Job drawing, mm, ordinate dimensions from the low corner. One solid piece. A direction names the side the tool comes from. Coordinates: 2 decimals unless noted, no trailing zeros. Loops run counter-clockwise (first coordinate to the right, second up) from the corner with the lowest first, then second, coordinate; pieces in that order, holes last. Notation, with made-up numbers: (54, 87.25) - (76, 87.25) arc R16 ccw to (76, 114.25) - close; hole circle Ø10 at (20, 34). An arc over 180 degrees is marked (long way). Use a Markdown table: item, result. Add a question column.
1) Probe probe 1 along Y at (x, z) = (11, 9.75); probe 2 along Z at (x, y) = (21.55, 11); probe 3 along Z at (x, y) = (14.25, 7.5). List the from-to ranges inside material, lowest first. Write a range as [from, to].
2) Band-saw the part on A-A (x = 11). Give the cut face in (y, z).
3) Band-saw the part on D-D (y = 16.75). Give the cut face in (x, z), plus the area to 3 significant figures.
4) Drop flat-ended pins along their axis: P1, Ø8, axis at x = 11, z = 8, coming from the +Y side; P2, Ø2, axis at y = 11.5, z = 4.5, coming from the +X side; P3, Ø6, axis at x = 11, y = 11, coming from the +Z side. Give the stop position or say it passes through.
5) Band-saw the part on C-C (z = 8). Give the cut face in (x, y), plus the area to 3 significant figures.
6) Tool access for the marked faces 4, 5, 6 and 7: list every direction of +Z, -Z, +X, -X, +Y, -Y with a clear straight run to the whole face (end or side of a thin tool).
7) Pull direction Z, two halves, no side cores. Call the marked faces 1, 2 and 3: +Z half, -Z half, draft (parallel to the pull), parting line (faces both ways), or undercut.
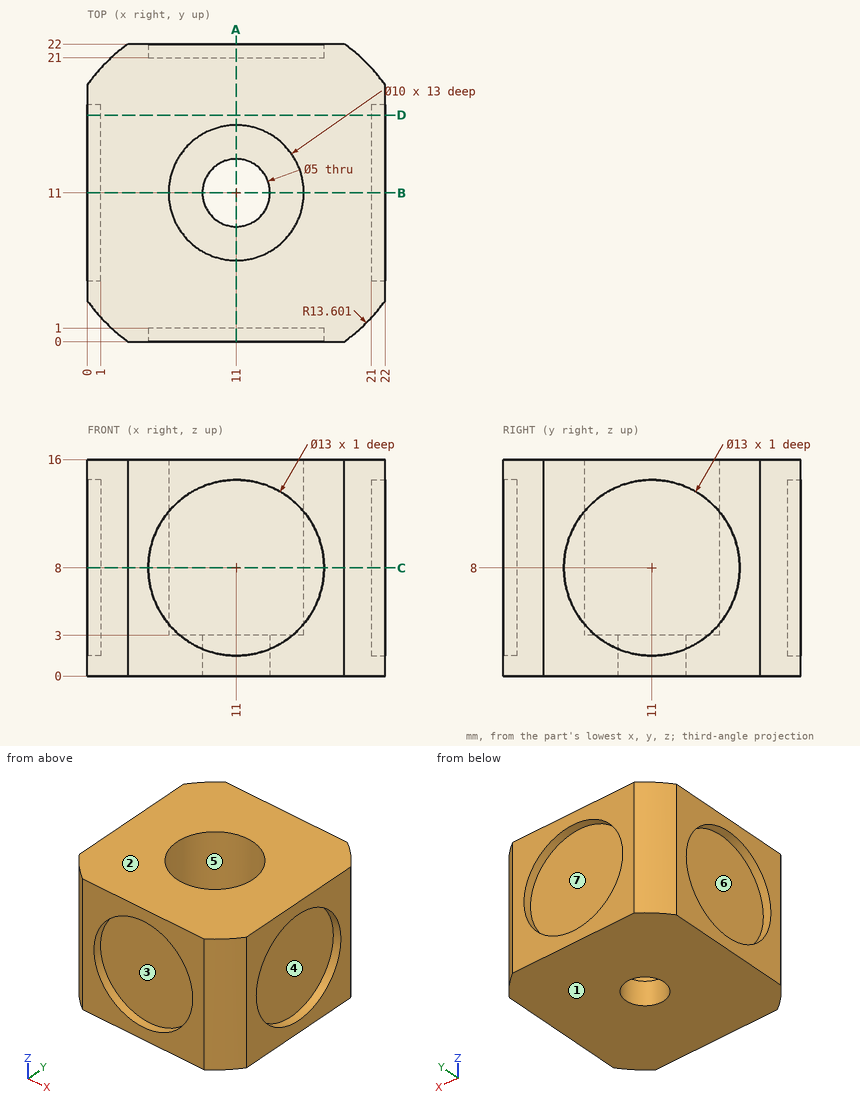
Answer block:
| question | item | result |
|---|---|---|
| 1 | probe 1 | [1, 6], [16, 21] |
| 1 | probe 2 | [0, 1.5], [14.5, 16] |
| 1 | probe 3 | [0, 3] |
| 2 | outline | (0, 0) - (8.5, 0) - (8.5, 3) - (6, 3) - (6, 16) - (0, 16) - (0, 14.5) - (1, 14.5) - (1, 1.5) - (0, 1.5) - close; (13.5, 0) - (22, 0) - (22, 1.5) - (21, 1.5) - (21, 14.5) - (22, 14.5) - (22, 16) - (16, 16) - (16, 3) - (13.5, 3) - close |
| 3 | outline | (0, 0) - (22, 0) - (22, 4.97) - (21, 4.97) - (21, 11.03) - (22, 11.03) - (22, 16) - (0, 16) - (0, 11.03) - (1, 11.03) - (1, 4.97) - (0, 4.97) - close |
| 3 | area | 340 mm2 |
| 4 | P1 | y = 21 |
| 4 | P2 | x = 21 |
| 4 | P3 | z = 3 |
| 5 | outline | (0, 3) arc R13.6 ccw to (3, 0) - (4.5, 0) - (4.5, 1) - (17.5, 1) - (17.5, 0) - (19, 0) arc R13.6 ccw to (22, 3) - (22, 4.5) - (21, 4.5) - (21, 17.5) - (22, 17.5) - (22, 19) arc R13.6 ccw to (19, 22) - (17.5, 22) - (17.5, 21) - (4.5, 21) - (4.5, 22) - (3, 22) arc R13.6 ccw to (0, 19) - (0, 17.5) - (1, 17.5) - (1, 4.5) - (0, 4.5) - close; hole circle Ø10 at (11, 11) |
| 5 | area | 337 mm2 |
| 6 | face 4 | +X |
| 6 | face 5 | +Z |
| 6 | face 6 | -X |
| 6 | face 7 | +Y |
| 7 | face 1 | -Z half |
| 7 | face 2 | +Z half |
| 7 | face 3 | undercut |
